Could you check a few things on this model? Use its own coordinates, in mm. A direction names the side the tool comes from. Give positions to 0.01 mm unless a question says otherwise; leave off trailing zeros. Write each loop counter-clockwise with the first axis right and the second up, starting at its lowest first coordinate (ties: lowest second). Pieces come first, ordered by that corner, then holes. Notation, with made-up numbers: M -21,58.25 L 31,58.25 A14 cw 31,84.25 Z; hole C 72.5,27 d10. An arc over 180 degrees is marked long. One line per item, written item: value.
```python
from build123d import *

# Parameters (mm, degrees)
EXTRUDE_1_DEPTH      = 2.2
EXTRUDE_2_DEPTH      = 3.25
SKETCH_3_W           = 50
SKETCH_3_H           = 10.05
EXTRUDE_3_DEPTH      = 3.25
CUT_EXTRUDE_1_DEPTH  = 30
EXTRUDE_4_REACH      = 56.389
SKETCH_6_R           = 5.025
SKETCH_8_R           = 1.675
SKETCH_8_R_2         = 0.84
CUT_EXTRUDE_3_DEPTH  = 55
SKETCH_9_W           = 28.473000816
SKETCH_9_H           = 14.532409192
CUT_EXTRUDE_4_DEPTH  = 3
EXTRUDE_5_DEPTH      = 2.45
SKETCH_11_W          = 12.614203935
SKETCH_11_H          = 10.05
EXTRUDE_6_DEPTH      = 3
SKETCH_12_W          = 36.628466797
SKETCH_12_H          = 15.348537224
CUT_EXTRUDE_5_DEPTH  = 10
SKETCH_13_W          = 5.35
SKETCH_13_H          = 5.35
CUT_EXTRUDE_6_DEPTH  = 14
SKETCH_14_R          = 1.1
CUT_EXTRUDE_7_DEPTH  = 14
SKETCH_15_R          = 1.1
CUT_EXTRUDE_8_DEPTH  = 10
SKETCH_16_R          = 1.625
EXTRUDE_7_DEPTH      = 5.7
SKETCH_17_W          = 19.923143876
SKETCH_17_H          = 15.083058075
CUT_EXTRUDE_9_DEPTH  = 3
SKETCH_18_R          = 1.675
SKETCH_18_R_2        = 1.6
CUT_EXTRUDE_10_DEPTH = 6
CUT_EXTRUDE_11_DEPTH = 10
EXTRUDE_8_DEPTH      = 9.5
EXTRUDE_9_DEPTH      = 15.2
SKETCH_23_W          = 14.793785908
SKETCH_23_H          = 11.59723546
CUT_EXTRUDE_12_DEPTH = 9
SKETCH_25_R          = 1.6
SKETCH_25_R_2        = 1.673969756
CUT_EXTRUDE_13_DEPTH = 20
FILLET_1_R           = 5
EXTRUDE_START        = 5
EXTRUDE_10_DEPTH     = 5
EXTRUDE_11_DEPTH     = 25.2


with BuildPart() as part:
    # 草图1 → 凸台-拉伸1 (new body)
    with BuildSketch(Plane.XY):
        with BuildLine():
            Line((1.539836705, 12.851012384), (15.55297303, 14.251012384))
            ThreePointArc((15.55297303, 14.251012384), (17.193415997, 16.063512384), (15.55297303, 17.876012384))
            Line((15.55297303, 17.876012384), (1.500532553, 18.901012384))
            ThreePointArc((1.500532553, 18.901012384), (0.527100583, 19.384612538), (-0.54702697, 19.551012384))
            Line((-0.54702697, 19.551012384), (-0.54702697, 20.901012384))
            Line((-0.54702697, 20.901012384), (19.51277613, 20.901012384))
            Line((19.51277613, 20.901012384), (41.45297303, 20.901012384))
            Line((41.45297303, 20.901012384), (41.45297303, 10.851012384))
            Line((41.45297303, 10.851012384), (-0.54702697, 10.851012384))
            Line((-0.54702697, 10.851012384), (-0.54702697, 12.201012384))
            ThreePointArc((-0.54702697, 12.201012384), (0.54584768, 12.367273294), (1.539836705, 12.851012384))
        make_face()
    extrude(amount=EXTRUDE_1_DEPTH)

    # 草图2 → 凸台-拉伸2 (add)
    with BuildSketch(Plane(origin=(0, 0, 0), x_dir=(-1, 0, 0), z_dir=(0, 0, -1))):
        Polygon((-19.51277613, 10.851012384), (-49.45297303, 10.851012384), (-49.45297303, 20.901012384), (-19.51277613, 20.901012384), (0.54702697, 20.901012384), (0.54702697, 10.851012384), align=None)
    extrude(amount=EXTRUDE_2_DEPTH)

    # 草图3 → 凸台-拉伸3 (add)
    with BuildSketch(Plane.XY.offset(2.2)):
        with Locations((24.45297303, 15.876012384)):
            Rectangle(SKETCH_3_W, SKETCH_3_H)
    extrude(amount=EXTRUDE_3_DEPTH)

    # 草图4 → 切除-拉伸1 (cut, symmetric)
    with BuildSketch(Plane.XY):
        with BuildLine():
            Line((-0.54702697, 19.551012384), (-2.235397712, 16.616091152))
            Line((-2.235397712, 16.616091152), (-1.110896638, 12.310548833))
            Line((-1.110896638, 12.310548833), (-0.54702697, 12.201012384))
            ThreePointArc((-0.54702697, 12.201012384), (0.54584768, 12.367273294), (1.539836705, 12.851012384))
            ThreePointArc((1.539836705, 12.851012384), (2.773180655, 15.88415254), (1.500532553, 18.901012384))
            ThreePointArc((1.500532553, 18.901012384), (0.527100583, 19.384612538), (-0.54702697, 19.551012384))
        make_face()
    extrude(amount=CUT_EXTRUDE_1_DEPTH, both=True, mode=Mode.SUBTRACT)

    # 凸台-拉伸4: up to this face of the body (flat: up to its plane)
    extrude_4_end = Plane(part.part.faces().sort_by_distance((25.407741746, 15.876338503, 5.45))[0])
    # 草图6 → 凸台-拉伸4 (add, up to the picked face)
    with BuildSketch(Plane(origin=(0, 0, -3.25), x_dir=(-1, 0, 0), z_dir=(0, 0, -1)), mode=Mode.PRIVATE) as extrude_4_sk1:
        with Locations(Location((-49.45297303, 15.876012384, 0), (0, 0, 90))):
            Circle(SKETCH_6_R)
    extrude_4_tool1 = split(extrude(extrude_4_sk1.sketch, amount=-EXTRUDE_4_REACH, mode=Mode.PRIVATE), bisect_by=extrude_4_end, keep=Keep.BOTH, mode=Mode.PRIVATE)
    add(extrude_4_tool1.solids().sort_by(Axis((49.452973, 15.876012, -3.25), (0, 0, 1)))[0])

    # 草图8 → 切除-拉伸3 (cut)
    with BuildSketch(Plane(origin=(0, 0, -3.25), x_dir=(-1, 0, 0), z_dir=(0, 0, -1))):
        with Locations((-49.45297303, 15.876012384)):
            Circle(SKETCH_8_R)
        with Locations(Location((-7.95297303, 15.856360308, 0), (0, 0, 180))):
            Circle(SKETCH_8_R_2)
    extrude(amount=-CUT_EXTRUDE_3_DEPTH, mode=Mode.SUBTRACT)

    # 草图9 → 切除-拉伸4 (cut)
    with BuildSketch(Plane(origin=(0, 0, -3.25), x_dir=(-1, 0, 0), z_dir=(0, 0, -1))):
        with Locations((-42.648638606, 15.039406696)):
            Rectangle(SKETCH_9_W, SKETCH_9_H)
    extrude(amount=-CUT_EXTRUDE_4_DEPTH, mode=Mode.SUBTRACT)

    # 草图10 → 凸台-拉伸5 (add)
    with BuildSketch(Plane(origin=(0, 0, 2.2), x_dir=(-1, 0, 0), z_dir=(0, 0, -1))):
        with BuildLine():
            Line((-49.45297303, 20.901012384), (-38.466384114, 20.901012384))
            Line((-38.466384114, 20.901012384), (-38.466384114, 10.851012384))
            Line((-38.466384114, 10.851012384), (-49.45297303, 10.851012384))
            ThreePointArc((-49.45297303, 10.851012384), (-46.217908976, 15.876012384), (-49.45297303, 20.901012384))
        make_face()
    extrude(amount=EXTRUDE_5_DEPTH)

    # 草图11 → 凸台-拉伸6 (add)
    with BuildSketch(Plane(origin=(0, 0, -3.25), x_dir=(-1, 0, 0), z_dir=(0, 0, -1))):
        with Locations((-32.625453647, 15.876012384)):
            Rectangle(SKETCH_11_W, SKETCH_11_H)
    extrude(amount=-EXTRUDE_6_DEPTH)

    # 草图12 → 切除-拉伸5 (cut)
    with BuildSketch(Plane(origin=(0, 0, -3.25), x_dir=(-1, 0, 0), z_dir=(0, 0, -1))):
        with Locations((-5.618322216, 15.103365543)):
            Rectangle(SKETCH_12_W, SKETCH_12_H)
    extrude(amount=-CUT_EXTRUDE_5_DEPTH, mode=Mode.SUBTRACT)

    # 草图13 → 切除-拉伸6 (cut)
    with BuildSketch(Plane.ZY.offset(-23.932555614)):
        with Locations((1.1, 16.124405573)):
            Rectangle(SKETCH_13_W, SKETCH_13_H)
    extrude(amount=-CUT_EXTRUDE_6_DEPTH, mode=Mode.SUBTRACT)

    # 草图14 → 切除-拉伸7 (cut)
    with BuildSketch(Plane(origin=(0, 20.901012384, 0), x_dir=(1, 0, 0), z_dir=(0, 1, 0))):
        with Locations(Location((30.538219594, -1.1, 0), (0, 0, 270))):
            Circle(SKETCH_14_R)
    extrude(amount=-CUT_EXTRUDE_7_DEPTH, mode=Mode.SUBTRACT)

    # 草图15 → 切除-拉伸8 (cut)
    with BuildSketch(Plane.XY.offset(5.45)):
        with Locations((36.879929969, 15.882801083)):
            Circle(SKETCH_15_R)
    extrude(amount=-CUT_EXTRUDE_8_DEPTH, mode=Mode.SUBTRACT)

    # 草图16 → 凸台-拉伸7 (add)
    with BuildSketch(Plane(origin=(0, 0, -0.25), x_dir=(-1, 0, 0), z_dir=(0, 0, -1))):
        with BuildLine():
            Line((-49.45297303, 20.901012384), (23.54702697, 20.901012384))
            ThreePointArc((23.54702697, 20.901012384), (28.57202697, 15.876012384), (23.54702697, 10.851012384))
            Line((23.54702697, 10.851012384), (-49.45297303, 10.851012384))
            Line((-49.45297303, 10.851012384), (-49.45297303, 20.901012384))
        make_face()
        with Locations((23.54702697, 15.876012384)):
            Circle(SKETCH_16_R, mode=Mode.SUBTRACT)
    extrude(amount=-EXTRUDE_7_DEPTH)

    # 草图17 → 切除-拉伸9 (cut)
    with BuildSketch(Plane(origin=(0, 0, -3.25), x_dir=(-1, 0, 0), z_dir=(0, 0, -1))):
        with Locations((-33.178239607, 16.007261263)):
            Rectangle(SKETCH_17_W, SKETCH_17_H)
    extrude(amount=-CUT_EXTRUDE_9_DEPTH, mode=Mode.SUBTRACT)

    # 草图18 → 切除-拉伸10 (cut)
    with BuildSketch(Plane(origin=(0, 0, -0.25), x_dir=(-1, 0, 0), z_dir=(0, 0, -1))):
        with Locations(Location((-49.45297303, 15.876012384, 0), (0, 0, 180))):
            Circle(SKETCH_18_R)
        with Locations((14.84318256, 15.876012384)):
            Circle(SKETCH_18_R_2)
        with BuildLine():
            Line((-31.661597205, 17.303258867), (8.461046927, 17.303258867))
            ThreePointArc((8.461046927, 17.303258867), (9.88829341, 15.876012384), (8.461046927, 14.448765901))
            Line((8.461046927, 14.448765901), (-31.661597205, 14.448765901))
            ThreePointArc((-31.661597205, 14.448765901), (-33.088843687, 15.876012384), (-31.661597205, 17.303258867))
        make_face()
    extrude(amount=-CUT_EXTRUDE_10_DEPTH, mode=Mode.SUBTRACT)

    # 草图19 → 切除-拉伸11 (cut)
    with BuildSketch(Plane(origin=(0, 0, -0.25), x_dir=(-1, 0, 0), z_dir=(0, 0, -1))):
        Polygon((12.697516125, 20.901012384), (-60.999534113, 39.375054119), (-58.738783937, -10.22846445), (12.697516125, 10.851012384), (10.156545193, 10.851012384), (10.156545193, 20.901012384), align=None)
    extrude(amount=-CUT_EXTRUDE_11_DEPTH, mode=Mode.SUBTRACT)

    # 草图21 → 凸台-拉伸8 (add)
    with BuildSketch(Plane.XY.offset(5.45)):
        with BuildLine():
            Line((-23.54702697, 20.901012384), (-12.697516125, 20.901012384))
            ThreePointArc((-12.697516125, 20.901012384), (-9.87974938, 15.876012384), (-12.697516125, 10.851012384))
            Line((-12.697516125, 10.851012384), (-23.54702697, 10.851012384))
            ThreePointArc((-23.54702697, 10.851012384), (-28.57202697, 15.876012384), (-23.54702697, 20.901012384))
        make_face()
    extrude(amount=EXTRUDE_8_DEPTH)

    # 草图22 → 凸台-拉伸9 (add)
    with BuildSketch(Plane(origin=(0, 0, -0.25), x_dir=(-1, 0, 0), z_dir=(0, 0, -1))):
        with BuildLine():
            Line((23.54702697, 20.901012384), (26.601137036, 16.368267617))
            Line((26.601137036, 16.368267617), (23.54702697, 10.851012384))
            ThreePointArc((23.54702697, 10.851012384), (26.480521945, 7.163010653), (28.555320944, 2.931940027))
            ThreePointArc((28.555320944, 2.931940027), (46.487809448, 16.320719833), (28.64667794, 29.830997223))
            ThreePointArc((28.64667794, 29.830997223), (26.554002303, 25.104940008), (23.54702697, 20.901012384))
        make_face()
    extrude(amount=-EXTRUDE_9_DEPTH)

    # 草图23 → 切除-拉伸12 (cut, symmetric)
    with BuildSketch(Plane(origin=(-10.156545193, 0, 0), x_dir=(0, 0, -1), z_dir=(1, 0, 0))):
        with Locations((-10.971714959, 15.6975909)):
            Rectangle(SKETCH_23_W, SKETCH_23_H)
    extrude(amount=CUT_EXTRUDE_12_DEPTH, both=True, mode=Mode.SUBTRACT)

    # 草图25 → 切除-拉伸13 (cut)
    with BuildSketch(Plane(origin=(0, 0, -0.25), x_dir=(-1, 0, 0), z_dir=(0, 0, -1))):
        with Locations((14.84318256, 15.876012384)):
            Circle(SKETCH_25_R)
        with Locations((23.54702697, 15.876012384)):
            Circle(SKETCH_25_R_2)
    extrude(amount=-CUT_EXTRUDE_13_DEPTH, mode=Mode.SUBTRACT)

    # 圆角1
    fillet_1_edges = [part.edges().sort_by_distance(p)[0] for p in [
        (-10.156545193, 10.851012384, 1.662411002),
        (-10.156545193, 20.901012384, 1.662411002),
    ]]
    fillet(fillet_1_edges, radius=FILLET_1_R)

    # 草图26 → 凸台-拉伸10 (add)
    with BuildSketch(Plane(origin=(0, 0, -0.25), x_dir=(-1, 0, 0), z_dir=(0, 0, -1)).offset(EXTRUDE_START)):
        with BuildLine():
            ThreePointArc((23.989483385, 21.41624515), (29.677771388, 15.903479456), (23.982335647, 10.398098659))
            ThreePointArc((23.982335647, 10.398098659), (26.300788095, 7.442479058), (28.078905502, 4.133520391))
            ThreePointArc((28.078905502, 4.133520391), (42.727883136, 16.096897132), (27.908169911, 27.848111056))
            ThreePointArc((27.908169911, 27.848111056), (26.188805201, 24.485968475), (23.989483385, 21.41624515))
        make_face()
    extrude(amount=-EXTRUDE_10_DEPTH)

    # 草图27 → 凸台-拉伸11 (add)
    with BuildSketch(Plane(origin=(0, 0, -5.25), x_dir=(-1, 0, 0), z_dir=(0, 0, -1))):
        with BuildLine():
            ThreePointArc((23.989483385, 21.41624515), (29.677771388, 15.903479456), (23.982335647, 10.398098659))
            ThreePointArc((23.982335647, 10.398098659), (26.300788095, 7.442479058), (28.078905502, 4.133520391))
            ThreePointArc((28.078905502, 4.133520391), (42.727883136, 16.096897132), (27.908169911, 27.848111056))
            ThreePointArc((27.908169911, 27.848111056), (26.188805201, 24.485968475), (23.989483385, 21.41624515))
        make_face()
    extrude(amount=-EXTRUDE_11_DEPTH)


solid = part.part
```
1) If we section it at C-C, the plane x = -35.5: Write out the boundary of the cut face in (y, z).
Outcome:
outline: M 2.7,-0.25 L 4.91,-0.25 L 4.91,-5.25 L 27.11,-5.25 L 27.11,-0.25 L 30.04,-0.25 L 30.04,14.95 L 27.11,14.95 L 27.11,19.95 L 4.91,19.95 L 4.91,14.95 L 2.7,14.95 Z
2) If we section it at B-B, the plane z = 12: Write out the boundary of the cut face in (x, y), then the cut area to 3 significant figures.
Outcome:
outline: M -28.65,29.83 A14 ccw long -28.56,2.93 A21.86 cw -23.55,10.85 L -19.16,10.85 L -19.16,20.9 L -23.55,20.9 A25.37 cw Z; hole C -23.55,15.88 d3.35
area: 537 mm^2
3) If we section it at D-D, the plane z = 1.25: Write out the boundary of the cut face in (x, y), then the cut area to 3 significant figures.
Outcome:
outline: M -28.65,29.83 A14 ccw long -28.56,2.93 A21.86 cw -23.55,10.85 L -15.16,10.85 A5 ccw -10.16,15.85 L -10.16,15.9 A5 ccw -15.16,20.9 L -23.55,20.9 A25.37 cw Z; hole C -23.55,15.88 d3.35; hole C -14.84,15.88 d3.2
area: 609 mm^2
4) We'd pull the mould along X, two halves only. Please class faces 6 (the face through (-21.875, 15.95, 7.244)), 7 (the face through (-20, 16, -0.25)), 8 (the face through (-11.66, 19.475, 1.689)), 9 (the face through (-15.581, 14.457, 1.636)): pulls with the +X half, pulls with the -X half, needs draft (parallel to the pull), parting line crosses it, or undercut.
Outcome:
face 6: undercut
face 7: needs draft
face 8: pulls with the +X half
face 9: undercut
5) On a 3-axis mill with a long thin cutter (end or side, diameter ignored), from which of +Z, -Z, +X, -X, +Y, -Y can I reach the whole of each face in a straight line? I mean faces 1 (the face through (-33, 16, 19.95)), 2 (the face through (-26, 16, 14.95)), 3 (the face through (-17, 16, 3.575)), 4 (the face through (-46.48, 15.96, 7.24)), 5 (the face through (-20, 20.901, 6)). Say none if no direction works.
Outcome:
face 1: +Z, +X, -X, +Y, -Y
face 2: +Z, +X
face 3: +Z, +X, +Y, -Y
face 4: +Z, -Z
face 5: +Z, -Z, +X, +Y
6) Please list where these lines run through material, in increasing order: L1, parallel to Z at x = -16, y = 12.75; L2, parallel to Z at x = -41, y = 6; L3, parallel to Y at x = -20, z = 8.5. Write a range as from..to.
Outcome:
L1: z = -0.25..3.57
L2: z = -0.25..14.95
L3: y = 10.85..20.9
7) I'm going to push flat-ended pins straight in: pin 1 (9 mm diameter, centred on x = -20, z = 3.5, fed in from -Y); pin 2 (3 mm diameter, centred on x = -26.5, y = 13.5, fed in from +Z); pin 3 (12 mm diameter, centred on x = -15.5, y = 17.5, fed in from -Z). Where does each tip first touch, or does it pass through?
Outcome:
pin 1: stops at y = 9.82
pin 2: stops at z = 14.95
pin 3: stops at z = -0.25
8) If we section it at A-A, the plane x = -16: Write out the boundary of the cut face in (y, z), then the cut area to 3 significant figures.
Outcome:
outline: M 10.85,-0.25 L 14.77,-0.25 L 14.77,3.57 L 10.85,3.57 Z; M 16.98,-0.25 L 20.9,-0.25 L 20.9,3.57 L 16.98,3.57 Z
area: 30.0 mm^2
